```python
from build123d import *

# Parameters (mm, degrees)
SKETCH1_W           = 80
SKETCH1_H           = 50
SKETCH1_R           = 5.5
SKETCH1_R_2         = 2.5
BOSS_EXTRUDE1_DEPTH = 12
SKETCH2_R           = 4.6
CUT_EXTRUDE1_DEPTH  = 1.55
SKETCH3_R           = 8.05
CUT_EXTRUDE2_DEPTH  = 4.5
SKETCH4_R           = 2.5
CUT_EXTRUDE3_DEPTH  = 11


with BuildPart() as part:
    # Sketch1 → Boss-Extrude1 (new body)
    with BuildSketch(Plane.XY):
        with Locations((40, 25)):
            Rectangle(SKETCH1_W, SKETCH1_H)
        with Locations((40, 32.4)):
            Circle(SKETCH1_R, mode=Mode.SUBTRACT)
        with Locations((10, 30)):
            Circle(SKETCH1_R_2, mode=Mode.SUBTRACT)
        with Locations((70, 30)):
            Circle(SKETCH1_R_2, mode=Mode.SUBTRACT)
        with Locations((30, 10)):
            Circle(SKETCH1_R_2, mode=Mode.SUBTRACT)
        with Locations((50, 10)):
            Circle(SKETCH1_R_2, mode=Mode.SUBTRACT)
        with Locations((16.4, 8.9)):
            Circle(SKETCH1_R_2, mode=Mode.SUBTRACT)
        with Locations((63.6, 8.9)):
            Circle(SKETCH1_R_2, mode=Mode.SUBTRACT)
    extrude(amount=BOSS_EXTRUDE1_DEPTH)

    # Sketch2 → Cut-Extrude1 (cut)
    with BuildSketch(Plane.XY.offset(12)):
        with Locations((10, 30)):
            Circle(SKETCH2_R)
        with Locations((70, 30)):
            Circle(SKETCH2_R)
        with Locations((30, 10)):
            Circle(SKETCH2_R)
        with Locations((50, 10)):
            Circle(SKETCH2_R)
    extrude(amount=-CUT_EXTRUDE1_DEPTH, mode=Mode.SUBTRACT)

    # Sketch3 → Cut-Extrude2 (cut)
    with BuildSketch(Plane(origin=(0, 0, 0), x_dir=(-1, 0, 0), z_dir=(0, 0, -1))):
        with Locations((-40, 32.4)):
            Circle(SKETCH3_R)
    extrude(amount=-CUT_EXTRUDE2_DEPTH, mode=Mode.SUBTRACT)

    # Sketch4 → Cut-Extrude3 (cut)
    with BuildSketch(Plane(origin=(0, 50, 0), x_dir=(1, 0, 0), z_dir=(0, 1, 0))):
        with Locations((50, -6)):
            Circle(SKETCH4_R)
        with Locations((30, -6)):
            Circle(SKETCH4_R)
    extrude(amount=-CUT_EXTRUDE3_DEPTH, mode=Mode.SUBTRACT)


solid = part.part
```
Source: CAD feature listing. Evaluate the final solid. Frame: model axes, mm. A direction names the side the tool comes from. Round coordinates to 2 decimals unless told otherwise and drop trailing zeros. Loops run counter-clockwise (first coordinate to the right, second up) from the corner with the lowest first, then second, coordinate; pieces in that order, holes last. Notation, with made-up numbers: M 23.5,13 L 60.5,13 A16 cw 60.5,25 Z; hole C 86,71.25 d8. An arc over 180 degrees is marked long. Use a Markdown table: item, result. Add a question column.
1. Contact query for flat-ended pins moving along their axis: P1, Ø6.5, axis at x = 70, y = 30, coming from the +Z side; P2, Ø13, axis at x = 40, y = 32.4, coming from the -Z side. Output: stop coordinate, or through.
2. Section query A-A on x = 30. Return the cut outline in (y, z).
3. Section query D-D on x = 10. Return the cut outline in (y, z), then the cut area to 3 significant figures.
4. Section query B-B on z = 6. Return the cut outline in (x, y).
5. Section query C-C on y = 8.9. Return the cut outline in (x, z) (3 decimals).
6. Line query: line 1 (X direction, y = 8, z = 7.5); line 2 (Y direction, x = 50, z = 11.25); line 3 (Z direction, x = 30, y = 44). Output: solid intervals per line, ascending.
7. Reachability of faces 5 (the flat face through (72, 28, 10.45)), 6 (the cylindrical face through (48.042, 32.754, 2.218)), 7 (the cylindrical face through (52.31, 44.58, 6.96)) from +Z, -Z, +X, -X, +Y, -Y: full face, straight path, thin tool, end or side. Return the list, or none.
8. Mould query, pull axis X, two halves, no side actions, for faces 1 (the flat face through (38, 27, 4.5)), 2 (the cylindrical face through (14.25, 28.24, 11.24)), 3 (the flat face through (39, 0, 6)), 4 (the flat face through (80, 25, 6)). Classes: pulls with the +X half, pulls with the -X half, needs draft (parallel to the pull), parting line crosses it, or undercut.
Reported:
| question | item | result |
|---|---|---|
| 1 | P1 | stops at z = 10.45 |
| 1 | P2 | stops at z = 4.5 |
| 2 | outline | M 0,0 L 7.5,0 L 7.5,10.45 L 5.4,10.45 L 5.4,12 L 0,12 Z; M 12.5,0 L 50,0 L 50,3.5 L 39,3.5 L 39,8.5 L 50,8.5 L 50,12 L 14.6,12 L 14.6,10.45 L 12.5,10.45 Z |
| 3 | outline | M 0,0 L 27.5,0 L 27.5,10.45 L 25.4,10.45 L 25.4,12 L 0,12 Z; M 32.5,0 L 50,0 L 50,12 L 34.6,12 L 34.6,10.45 L 32.5,10.45 Z |
| 3 | area | 533 mm² |
| 4 | outline | M 0,0 L 80,0 L 80,50 L 52.5,50 L 52.5,39 L 47.5,39 L 47.5,50 L 32.5,50 L 32.5,39 L 27.5,39 L 27.5,50 L 0,50 Z; hole C 10,30 d5; hole C 16.4,8.9 d5; hole C 30,10 d5; hole C 40,32.4 d11; hole C 50,10 d5; hole C 63.6,8.9 d5; hole C 70,30 d5 |
| 5 | outline | M 0,0 L 13.9,0 L 13.9,12 L 0,12 Z; M 18.9,0 L 27.755,0 L 27.755,10.45 L 25.533,10.45 L 25.533,12 L 18.9,12 Z; M 32.245,0 L 47.755,0 L 47.755,10.45 L 45.533,10.45 L 45.533,12 L 34.467,12 L 34.467,10.45 L 32.245,10.45 Z; M 52.245,0 L 61.1,0 L 61.1,12 L 54.467,12 L 54.467,10.45 L 52.245,10.45 Z; M 66.1,0 L 80,0 L 80,12 L 66.1,12 Z |
| 6 | line 1 | x = 0 to 14.07, 18.73 to 28.5, 31.5 to 48.5, 51.5 to 61.27, 65.93 to 80 |
| 6 | line 2 | y = 0 to 5.4, 14.6 to 50 |
| 6 | line 3 | z = 0 to 3.5, 8.5 to 12 |
| 7 | face 5 | +Z |
| 7 | face 6 | -Z |
| 7 | face 7 | +Y |
| 8 | face 1 | undercut |
| 8 | face 2 | undercut |
| 8 | face 3 | needs draft |
| 8 | face 4 | pulls with the +X half |
